from build123d import *

# Parameters (mm, degrees)
EXTRUDE_1_DEPTH          = 60
CUT_EXTRUDE_1_DEPTH      = 40
CUT_EXTRUDE_1_DEPTH_BACK = 40
SKETCH_2_R               = 7.25
SKETCH_3_R               = 8
SKETCH_3_R_2             = 6
EXTRUDE_2_DEPTH          = 1
CUT_EXTRUDE_2_REACH      = 75.103
SKETCH_4_R               = 2


with BuildPart() as part:
    # 草图1 → 凸台-拉伸1 (new body)
    with BuildSketch(Plane.XY):
        Polygon((0, 0), (0, 40), (8, 40), (8, 41.2), (-12, 41.2), (-12, 40), (-4, 40), (-4, 0), align=None)
    extrude(amount=EXTRUDE_1_DEPTH)

    # 草图2 → 切除-拉伸1 (cut, two sides: drawn at the far end of the back side and taken through both)
    with BuildSketch(Plane(origin=(0, 0, 0), x_dir=(0, 0, -1), z_dir=(1, 0, 0)).offset(-CUT_EXTRUDE_1_DEPTH_BACK)):
        with BuildLine():
            ThreePointArc((-19.604755263, 6.005094925), (-23.997453078, 1.609166037), (-30, 0))
            Line((-30, 0), (0, 0))
            Line((0, 0), (0, 40))
            Line((0, 40), (-19.604755263, 6.005094925))
        make_face()
        with BuildLine():
            Line((-40.395244737, 6.005094925), (-60, 40))
            Line((-60, 40), (-60, 0))
            Line((-60, 0), (-30, 0))
            ThreePointArc((-30, 0), (-36.002546922, 1.609166037), (-40.395244737, 6.005094925))
        make_face()
        with Locations(Location((-30, 12, 0), (0, 0, 180))):
            Circle(SKETCH_2_R)
        with BuildLine():
            Line((-51.166010489, 41.2), (-8.833989511, 41.2))
            ThreePointArc((-8.833989511, 41.2), (-30, 25.2), (-51.166010489, 41.2))
        make_face()
    extrude(amount=CUT_EXTRUDE_1_DEPTH + CUT_EXTRUDE_1_DEPTH_BACK, mode=Mode.SUBTRACT)

    # 草图3 → 凸台-拉伸2 (add)
    with BuildSketch(Plane.ZY.offset(4)):
        with Locations(Location((30, 12, 0), (0, 0, 90))):
            Circle(SKETCH_3_R)
        with Locations(Location((30, 12, 0), (0, 0, 270))):
            Circle(SKETCH_3_R_2, mode=Mode.SUBTRACT)
    extrude(amount=EXTRUDE_2_DEPTH)

    # 草图4 → 切除-拉伸2 (cut, up to next)
    with BuildSketch(Plane.XZ.offset(-40), mode=Mode.PRIVATE) as cut_extrude_2_sk1:
        with Locations((-8.5, 4)):
            Circle(SKETCH_4_R)
    cut_extrude_2_tool1 = extrude(cut_extrude_2_sk1.sketch, amount=-CUT_EXTRUDE_2_REACH, mode=Mode.PRIVATE) & part.part
    # 草图4 → 切除-拉伸2 (cut, up to next)
    with BuildSketch(Plane.XZ.offset(-40), mode=Mode.PRIVATE) as cut_extrude_2_sk2:
        with Locations((4.5, 4)):
            Circle(SKETCH_4_R)
    cut_extrude_2_tool2 = extrude(cut_extrude_2_sk2.sketch, amount=-CUT_EXTRUDE_2_REACH, mode=Mode.PRIVATE) & part.part
    # 草图4 → 切除-拉伸2 (cut, up to next)
    with BuildSketch(Plane.XZ.offset(-40), mode=Mode.PRIVATE) as cut_extrude_2_sk3:
        with Locations((-8.5, 56)):
            Circle(SKETCH_4_R)
    cut_extrude_2_tool3 = extrude(cut_extrude_2_sk3.sketch, amount=-CUT_EXTRUDE_2_REACH, mode=Mode.PRIVATE) & part.part
    # 草图4 → 切除-拉伸2 (cut, up to next)
    with BuildSketch(Plane.XZ.offset(-40), mode=Mode.PRIVATE) as cut_extrude_2_sk4:
        with Locations((4.5, 56)):
            Circle(SKETCH_4_R)
    cut_extrude_2_tool4 = extrude(cut_extrude_2_sk4.sketch, amount=-CUT_EXTRUDE_2_REACH, mode=Mode.PRIVATE) & part.part
    add(cut_extrude_2_tool1.solids().sort_by_distance((-8.5, 40, 4))[0], mode=Mode.SUBTRACT)
    add(cut_extrude_2_tool2.solids().sort_by_distance((4.5, 40, 4))[0], mode=Mode.SUBTRACT)
    add(cut_extrude_2_tool3.solids().sort_by_distance((-8.5, 40, 56))[0], mode=Mode.SUBTRACT)
    add(cut_extrude_2_tool4.solids().sort_by_distance((4.5, 40, 56))[0], mode=Mode.SUBTRACT)


solid = part.part
The listing builds one solid part. Answer for the finished solid, in the listing's coordinates (mm). A direction names the side the tool comes from. Round coordinates to 2 decimals unless told otherwise and drop trailing zeros. Write each loop counter-clockwise with the first axis right and the second up, starting at its lowest first coordinate (ties: lowest second). Pieces come first, ordered by that corner, then holes. Notation, with made-up numbers: M 24,15 L 70,15 A6 ccw 70,21 Z; hole C 41.5,-19.5 d10. An arc over 180 degrees is marked long. Write each question's results on one line, items separated by ' | '. Start each with the question number.
Item 1: For faces 1 (the face through (-4.493, 10.959, 22.068)), 2 (the face through (-10.1, 40.6, 2.8)), 3 (the face through (-7, 40, 6)), 4 (the face through (-12, 41, 5)), 5 (the face through (0, 21, 30)), determine the directions among +Z, -Z, +X, -X, +Y, -Y from which every point of the face is accessible in a straight line to the end or side of a thin tool.
Item 2: Straight lines are drawn through the part: L1, parallel to Z at x = -8.5, y = 40.8; L2, parallel to X at y = 18, z = 17; L3, parallel to Y at x = 3.5, z = 52. For each, find the intervals that lie inside material, in ascending order. Write a range as [from, to].
Item 3: For a pull along Z with two mould halves and no side action, classify faces 6 (the face through (-2.028, 11.681, 22.757)), 7 (the face through (-7, 40, 54)), 8 (the face through (-2, 41, 60)), 9 (the face through (-8.76, 40.592, 57.983)) as pulls with the +Z half, pulls with the -Z half, needs draft (parallel to the pull), parting line crosses it, or undercut.
Item 4: A cutting plane is placed at A-A on y = 26.5. Write down the section's boundary in (x, z), and give its area (3 significant figures).
Item 5: A cutting plane is placed at B-B on x = -8.5. Write down the section's boundary in (y, z).
Item 6: Flat-ended cylindrical pins translate along their axes: pin 1 Ø1 at (y, z) = (28, 52) entering from +X; pin 2 Ø12 at (y, z) = (24, 26) entering from -X; pin 3 Ø12 at (x, z) = (-5, 37.5) entering from +Y. Find the tip coordinate at first contact, or state that the pin passes through.
Item 7: A cutting plane is placed at D-D on z = 56. Write down the section's boundary in (x, y).
Item 8: A cutting plane is placed at C-C on z = 35. Write down the section's boundary in (x, y) (3 decimals).
Check sheet entries:
1) face 1: -X | face 2: +Y, -Y | face 3: +Z, -Z, -X, -Y | face 4: +Z, -Z, -X, +Y, -Y | face 5: +Z, -Z, +X, -Y
2) L1: [0, 2], [6, 8.95], [51.05, 54], [58, 60] | L2: [-4, 0] | L3: [40, 41.2]
3) face 6: undercut | face 7: needs draft | face 8: pulls with the +Z half | face 9: undercut
4) outline: M -4,7.79 L 0,7.79 L 0,22.55 L -4,22.55 Z; M -4,37.45 L 0,37.45 L 0,52.21 L -4,52.21 Z | area: 118 mm²
5) outline: M 40,0 L 41.2,0 L 41.2,2 L 40,2 Z; M 40,6 L 41.2,6 L 41.2,8.83 A22 cw 40,9.21 Z; M 40,50.79 A22 cw 41.2,51.17 L 41.2,54 L 40,54 Z; M 40,58 L 41.2,58 L 41.2,60 L 40,60 Z
6) pin 1: x = 0 | pin 2: x = -5 | pin 3: y = 29.76
7) outline: M -12,40 L -10.5,40 L -10.5,41.2 L -12,41.2 Z; M -6.5,40 L -4,40 L -4,33.06 L 0,33.06 L 0,40 L 2.5,40 L 2.5,41.2 L -6.5,41.2 Z; M 6.5,40 L 8,40 L 8,41.2 L 6.5,41.2 Z
8) outline: M -5,5.755 L -4,5.755 L -4,1.091 L 0,1.091 L 0,6.75 L -4,6.75 L -4,8.683 L -5,8.683 Z; M -5,15.317 L -4,15.317 L -4,17.25 L 0,17.25 L 0,25.776 L -4,25.776 L -4,18.245 L -5,18.245 Z
